Autodesk Inventor part; units mm, degrees
ref_plane "Work Plane1" through (1.525, 0, 0) normal (0, 0, 1) x (1, 0, 0)
ref_plane "YZ Plane" through (0, 0, 0) normal (1, 0, 0) x (0, 1, 0)
ref_plane "XZ Plane" through (0, 0, 0) normal (0, 1, 0) x (-1, 0, 0)
sketch "Sketch1" plane through (0, 0, 0) normal (0, 0, 1) x (1, 0, 0)
  line L0 (0, 7.1374) -> (0, 4.7625)
  line L1 (101.6, 4.7625) -> (127, 4.7625)
  line L2 (127, 4.7625) -> (127, 0)
  line L3 (127, 0) -> (-0.6351, 0)
  line L4 (-26.1621, 0) -> (152.527, 0)
  line L5 (-0.6351, 0) -> (-0.6351, 7.1374)
  line L6 (-0.6351, 7.1374) -> (0, 7.1374)
  line L7 (101.6, 4.7625) -> (90.4747, 4.7625)
  line L8 (90.4747, 4.7625) -> (0, 4.7625)
  line L9 (0, -1.4275) -> (0, 8.5649)
  dimension "d0" = 127
  dimension "d1" = 25.4
  dimension "d2" = 9.525
  dimension "d9" = 0.6351
  dimension "d10" = 14.2748
  dimension "d13" = 11.1253
  dimension "d14" = 9.525
revolve "Body" add sketch "Sketch1" angle 360 about axis through (127, 0, 0) along (-1, 0, 0)
sketch "Sketch2" plane through (-0.6351, 0, 0) normal (-1, 0, 0) x (0, 0, 1)
  line L0 (0, 8.2416) -> (7.1374, 4.1208)
  line L1 (7.1374, 4.1208) -> (7.1374, -4.1208)
  line L2 (7.1374, -4.1208) -> (0, -8.2416)
  line L3 (0, -8.2416) -> (-7.1374, -4.1208)
  line L4 (-7.1374, -4.1208) -> (-7.1374, 4.1208)
  line L5 (-7.1374, 4.1208) -> (0, 8.2416)
  point P0 (0, 0)
  point P1 (0, 0)
  dimension "d11" = 14.2748
extrude "Head" add sketch "Sketch2" along normal blind 5.5372
sketch "Sketch4" plane through (0, 0, 0) normal (0, 0, 1) x (1, 0, 0)
  line L0 (-6.1723, 7.1374) -> (-6.1723, 8.2416)
  line L1 (-6.1723, 8.2416) -> (-5.5348, 8.2416)
  line L2 (-5.5348, 8.2416) -> (-6.1723, 7.1374)
  line L3 (-7.2797, 0) -> (0.4723, 0)
  line L4 (-0.6351, 8.2416) -> (-6.1723, 8.2416)
  line L5 (-6.1723, 4.1208) -> (-6.1723, 8.2416)
  dimension "d5" = 30
  dimension "d19" = 14.2748
revolve "Chamfer1" cut sketch "Sketch4" angle 360 about axis through (-10, 0, 0) along (1, 0, 0)
thread "Thread"
chamfer "Chamfer2" distance 0.9738 distance2 0.9739 1 edges at (127, -4.7625, 0) measured on face at (127, -1.1883, 1.0527)
ref_plane "Work Plane1" through (1.525, 0, 0) normal (0, 0, 1) x (1, 0, 0)
equation "\"d0\" = NLG"
equation "\"d1\" = GEL"
equation "\"d2\" = GD"
equation "\"d10\" = SD2"
equation "\"d14\" = BDM"
equation "\"d11\" = SW"
equation "\"d3\" = KOH - SD"
equation "\"d5\" = ANG1"
equation "\"d19\" = SW0"
equation "\"d15\" = GEL"
equation "\"d6\" = -0.5 * SPD + 0.5 * GD"
equation "\"NLG\" = 127"
equation "\"GD\" = 9.525"
equation "\"BDM\" = 9.525"
equation "\"KOH\" = 6.1722"
equation "\"GEL\" = 25.4"
equation "\"SW\" = 14.2748"
equation "\"SW0\" = SW"
equation "\"SPD\" = GD1"
equation "\"SD2\" = SW"
equation "\"SD\" = 0.635"
equation "\"ANG1\" = 30deg"
equation "\"GAL\" = 11.1252"
equation "\"GUL\" = 0.97384"
equation "\"RR\" = 0.381"
equation "\"WFT\" = SD"
equation "\"GD1\" = 7.57733"
equation "\"THREADDIA\" = 9.525"
equation "\"SDH\" = SW"
equation "\"SDHG\" = 90.4748"
equation "\"TOA\" = 30deg"
equation "\"FAWI\" = 45deg"
equation "\"NND\" = 9.525"
equation "\"E0\" = 16.48739"
properties part number "AS 2465 - 3/8 x 5  UNC" material "Steel, Mild"
Verification items for the finished model (mm, model axes). A direction names the side the tool comes from. Round coordinates to 2 decimals unless told otherwise and drop trailing zeros. Order: outer loops, then holes, each group sorted by start corner. A loop starts at its lowest first (then second) coordinate and runs counter-clockwise, first axis right, second up. Notation, with made-up numbers: (32.5, 30) -> (56.5, 30) arc R27 cw to (56.5, 56) -> close; hole circle Ø8 at (-28.75, -36). An arc over 180 degrees is marked (long way). Put each result on its own line as item: value. Start each with the question number.
(1) Section check A-A (x = 37). Enter the section's corners in (y, z) (1 decimal).
(2) Depth check by flat-ended pin: pin 1 Ø6 at (x, z) = (65, -1.5) entering from -Y; pin 2 Ø6 at (x, z) = (35, -1.5) entering from +Y; pin 3 Ø2.5 at (y, z) = (-5, -2.5) entering from +X. Enter the tip coordinate at first touch or a pass-through.
(3) Material ranges on line 1 along X through (y, z) = (-2, 6); line 2 along X through (y, z) = (1.75, 3.5); line 3 along Z through (x, y) = (113.5, 4), recorded low to high.
(4) Tool access check on faces 1 (the face through (-0.635, 7.5, -0.6)), 2 (the face through (127, 0, 0)), 3 (the face through (-0.635, -7.5, -0.6)), 4 (the face through (63.9, -3.78, -2.9)). Record the directions out of +Z, -Z, +X, -X, +Y, -Y that give a thin tool (end or side, any length) a straight path to the whole face; none if there is none.
Completed:
1. outline: circle Ø9.5 at (0, 0)
2. pin 1: stops at y = -4.76
2. pin 2: stops at y = 4.76
2. pin 3: stops at x = 126.45
3. line 1: x = -6.17 to 0
3. line 2: x = -6.17 to 126.88
3. line 3: z = -2.58 to 2.58
4. face 1: +X, +Y
4. face 2: +Z, -Z, +X, +Y, -Y
4. face 3: +X, -Y
4. face 4: +X
